Answer from the drawing. Dimensions are ordinates in mm from the lowest x, y and z of the part. A direction names the side the tool comes from. Give positions to 0.01 mm unless a question says otherwise; leave off trailing zeros. Loops run counter-clockwise (first coordinate to the right, second up) from the corner with the lowest first, then second, coordinate; pieces in that order, holes last. Notation, with made-up numbers: (37, 78) - (49, 78) arc R15 ccw to (49, 82) - close; hole circle Ø3 at (23.5, 42). An arc over 180 degrees is marked (long way). One line per item, written item: value.
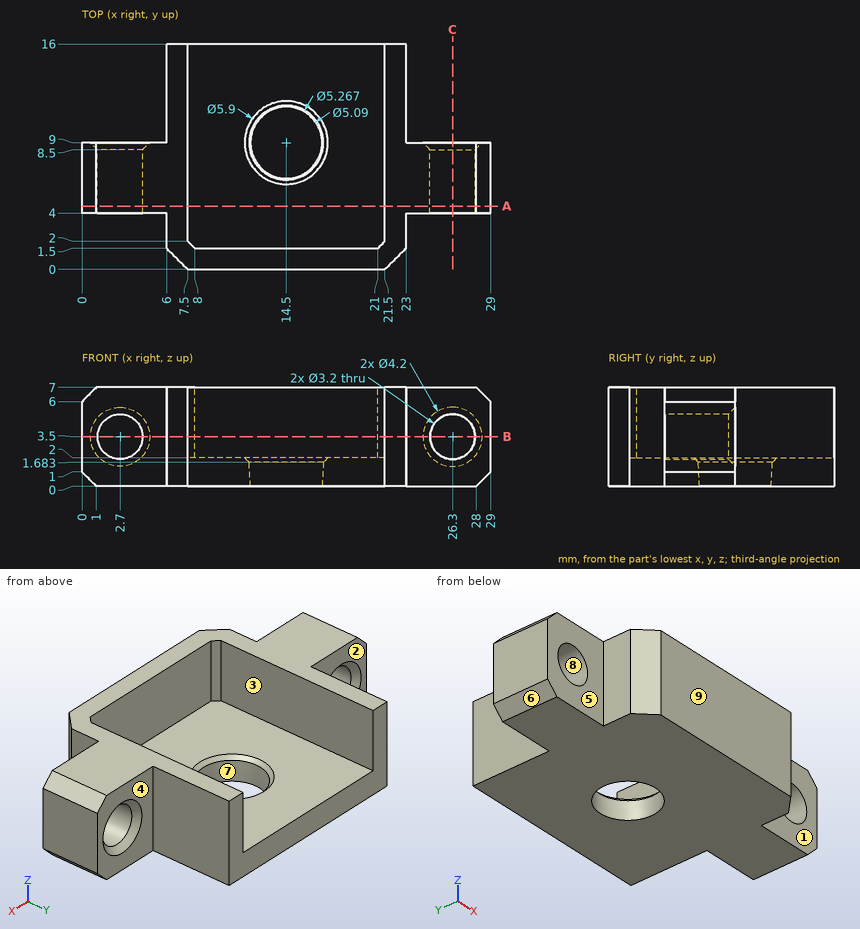
1. Flat-ended cylindrical pins translate along their axes: pin 1 Ø1.5 at (x, y) = (5, 13.5) entering from +Z; pin 2 Ø3.5 at (x, z) = (2.7, 3.5) entering from -Y; pin 3 Ø1.2 at (y, z) = (2.5, 5) entering from -X; pin 4 Ø1.5 at (x, z) = (19, 3) entering from -Y. Find the tip coordinate at first contact, or state that the pin passes through.
Output:
pin 1: passes through
pin 2: stops at y = 4
pin 3: stops at x = 6
pin 4: stops at y = 0
2. For the marked faces 1, 2, 3, 4 and 5, determine the directions among +Z, -Z, +X, -X, +Y, -Y from which every point of the face is accessible in a straight line to the end or side of a thin tool.
Output:
face 1: +Z, -Z, +X, -Y
face 2: +Z, -Z, -X, +Y
face 3: +Z, +Y
face 4: +Z, -Z, +X, +Y
face 5: +Z, -Z, -X, -Y
3. Section A-A (y = 4.5) is taken. Write down the section's boundary in (x, z), and give its area (3 significant figures).
Output:
outline: (0, 1) - (1, 0) - (28, 0) - (29, 1) - (29, 6) - (28, 7) - (21.5, 7) - (21.5, 2) - (7.5, 2) - (7.5, 7) - (1, 7) - (0, 6) - close; hole circle Ø3.2 at (2.7, 3.5); hole circle Ø3.2 at (26.3, 3.5)
area: 115 mm²
4. Find the intervals of material crossed by line 1 along X through (y, z) = (6.6, 3.5); line 2 along Z through (x, y) = (26.3, 5.6); line 3 along Y through (x, z) = (14.75, 6.5), in increasing order.
Output:
line 1: x = 0 to 1.1, 4.3 to 7.5, 21.5 to 24.7, 27.9 to 29
line 2: z = 0 to 1.9, 5.1 to 7
line 3: y = 0 to 1.5
5. The mould has two halves that part along X. Classify the marked faces 6, 7, 8 and 9: released by +X, released by -X, zero draft, split by the parting line, or undercut.
Output:
face 6: released by -X
face 7: undercut
face 8: undercut
face 9: zero draft
6. Section B-B (z = 3.5) is taken. Count the separate pieces of the cut face and the enclosed holes in it.
Output:
separate pieces: 3
enclosed holes: 0
7. Section C-C (x = 26.3) is taken. Write down the section's boundary in (y, z).
Output:
outline: (4, 0) - (9, 0) - (9, 1.4) - (8.5, 1.9) - (4, 1.9) - close; (4, 5.1) - (8.5, 5.1) - (9, 5.6) - (9, 7) - (4, 7) - close
